CAD build for the part. Positions are in the model's coordinates, mm. Face numbers are marked on the shaded views. Round coordinates to 2 decimals unless told otherwise and drop trailing zeros. Write each loop counter-clockwise with the first axis right and the second up, starting at its lowest first coordinate (ties: lowest second). Pieces come first, ordered by that corner, then holes. Notation, with made-up numbers: (-16, 20) - (10, 20) arc R18 cw to (10, 42) - close; hole circle Ø7 at (32, 70). An arc over 180 degrees is marked (long way). Answer in a Markdown table with one row per item.
```python
from build123d import *

# Parameters (mm, degrees)
BOSS_EXTRUDE1_DEPTH = 8
CHAMFER1_SIZE       = 5


with BuildPart() as part:
    # Sketch1 → Boss-Extrude1 (new body)
    with BuildSketch(Plane(origin=(0, 0, 0), x_dir=(1, 0, 0), z_dir=(0, 1, 0))):
        Polygon((-22.9, 0), (-12.9, 0), (-12.9, 60), (12.9, 60), (12.9, 0), (22.9, 0), (22.9, 70), (-22.9, 70), align=None)
    extrude(amount=BOSS_EXTRUDE1_DEPTH)

    # Chamfer1
    chamfer1_edges = [part.edges().sort_by_distance(p)[0] for p in [
        (-12.9, 8, -30),
        (0, 8, -60),
        (12.9, 8, -30),
    ]]
    chamfer(chamfer1_edges, length=CHAMFER1_SIZE)


solid = part.part
```
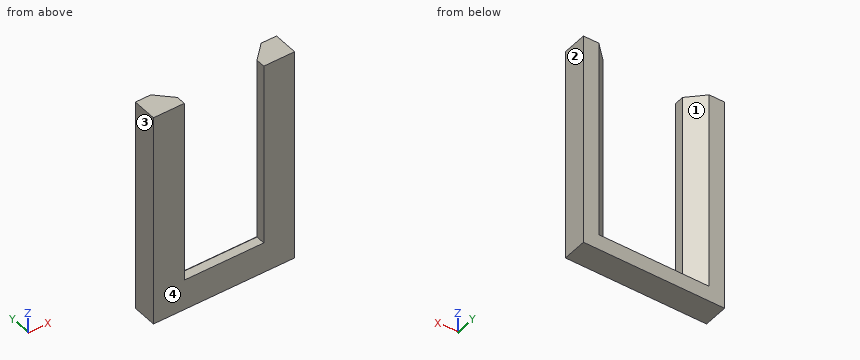
Q1. Saw through at D-D on y = 1.75. List the corners of the cut face in (x, z).
Computed:
| item | result |
|---|---|
| outline | (-22.9, -70) - (22.9, -70) - (22.9, 0) - (12.9, 0) - (12.9, -60) - (-12.9, -60) - (-12.9, 0) - (-22.9, 0) - close |
Q2. Saw through at B-B on y = 6.75. List the corners of the cut face in (x, z), then the cut area to 3 significant figures.
Computed:
| item | result |
|---|---|
| outline | (-22.9, -70) - (22.9, -70) - (22.9, 0) - (16.65, 0) - (16.65, -63.75) - (-16.65, -63.75) - (-16.65, 0) - (-22.9, 0) - close |
| area | 1,080 mm2 |
Q3. Saw through at A-A on z = -44. List the corners of the cut face in (x, y), then the cut area to 3 significant figures.
Computed:
| item | result |
|---|---|
| outline | (-22.9, 0) - (-12.9, 0) - (-12.9, 3) - (-17.9, 8) - (-22.9, 8) - close; (12.9, 0) - (22.9, 0) - (22.9, 8) - (17.9, 8) - (12.9, 3) - close |
| area | 135 mm2 |
Q4. Pull direction X, two halves, no side cores. Call the marked faces 1, 2, 3 and 4: released by +X, released by -X, zero draft, split by the parting line, or undercut.
Computed:
| item | result |
|---|---|
| face 1 | undercut |
| face 2 | released by +X |
| face 3 | released by -X |
| face 4 | zero draft |
Q5. Saw through at C-C on x = 15.5. List the corners of the cut face in (y, z), then the cut area to 3 significant figures.
Computed:
| item | result |
|---|---|
| outline | (0, -70) - (8, -70) - (8, -65) - (5.6, -62.6) - (5.6, 0) - (0, 0) - close |
| area | 407 mm2 |
Q6. Flat gauge pins, fed straight in: pin 1 (3.5 mm diameter, centred on x = -0.5, y = 1.5, fed in from +Z); pin 2 (2 mm diameter, centred on x = 16.5, z = -50.5, fed in from +Y); pin 3 (10 mm diameter, centred on x = 7, z = -7.5, fed in from -Y). Where does each tip first touch, or does it go through?
Computed:
| item | result |
|---|---|
| pin 1 | stops at z = -60 |
| pin 2 | stops at y = 7.6 |
| pin 3 | passes through |
Q7. Drill centre lines: line 1 (X direction, y = 1, z = -56); line 2 (X direction, y = 3.25, z = -50); line 3 (Z direction, x = -5, y = 1). Where is each one in solid material? Low to high.
Computed:
| item | result |
|---|---|
| line 1 | x = -22.9 to -12.9, 12.9 to 22.9 |
| line 2 | x = -22.9 to -13.15, 13.15 to 22.9 |
| line 3 | z = -70 to -60 |
